Autodesk Inventor part; units mm, degrees
ref_plane "YZ Plane" through (0, 0, 0) normal (1, 0, 0) x (0, 1, 0)
ref_plane "XZ Plane" through (0, 0, 0) normal (0, 1, 0) x (-1, 0, 0)
ref_plane "XY Plane" through (0, 0, 0) normal (0, 0, 1) x (1, 0, 0)
sketch "Sketch1" plane through (0, 0, 0) normal (0, 1, 0) x (-1, 0, 0)
  line L0 (-12.7, -12.7) -> (12.7, -12.7)
  line L1 (12.7, -12.7) -> (12.7, 12.7)
  line L2 (12.7, 12.7) -> (-12.7, 12.7)
  line L3 (-12.7, 12.7) -> (-12.7, -12.7)
  line L4 (-12.7, -12.7) -> (12.7, 12.7) construction
  line L5 (12.7, -12.7) -> (-12.7, 12.7) construction
  line L6 (9.525, 9.525) -> (9.525, -9.525)
  line L7 (9.525, -9.525) -> (-9.525, -9.525)
  line L8 (-9.525, -9.525) -> (-9.525, 9.525)
  line L9 (-9.525, 9.525) -> (9.525, 9.525)
  point P0 (0, 0)
  dimension "d0" = 25.4
  dimension "d1" = 25.4
  dimension "d2" = 3.175
extrude "Extrusion1" add sketch "Sketch1" along normal mid plane 711.2
sketch "Sketch2" plane through (-12.7, 355.6, 12.7) normal (0, 0, 1) x (1, 0, 0)
  line L0 (0, 0) -> (25.4, 0)
  line L1 (0, 0) -> (25.4, -25.4)
  line L2 (25.4, -711.2) -> (25.4, 0)
  circle A0 centre (12.7, -31.75) radius 3.2512
  circle A1 centre (12.7, -50.8) radius 3.2512
  line L3 (0, -711.2) -> (0, 0)
  line L4 (0, -355.6) -> (25.4, -355.6) construction
  line L5 (0, -711.2) -> (25.4, -711.2)
  line L6 (0, -711.2) -> (25.4, -685.8)
  circle A2 centre (12.7, -679.45) radius 3.2512
  circle A3 centre (12.7, -660.4) radius 3.2512
  circle A4 centre (12.7, -12.7) radius 3.2512
  circle A5 centre (12.7, -698.5) radius 3.2512
  point P0 (12.7, -355.6)
  point P1 (12.7, 0)
  point P2 (12.7, -711.2)
  point P3 (14.9989, -14.9989)
  point P4 (10.4011, -10.4011)
  point P5 (14.9989, -696.2011)
  point P6 (10.4011, -700.7989)
  dimension "d5" = 25.4
  dimension "d6" = 6.5024
  dimension "d7" = 31.75
  dimension "d8" = 19.05
extrude "Extrusion2" cut sketch "Sketch2" against normal blind 711.2 contours L0 L2 L1 A4 | A4 L1 | L1 A4 | L6 A5 L2 L5 | A5 L6 | L6 A5 | A0 | A1 | A2 | A3
sketch "Sketch4" plane through (-12.7, -355.6, 12.7) normal (0, 0, 1) x (1, 0, 0)
  line L0 (0, 0) -> (0, 711.2) construction
  line L1 (0, 355.6) -> (25.4, 355.6) construction
  line L2 (25.4, 25.4) -> (25.4, 685.8) construction
  circle A0 centre (12.7, 171.45) radius 3.2512
  circle A1 centre (12.7, 539.75) radius 3.2512
  point P0 (12.7, 355.6)
  dimension "d23" = 6.5024
  dimension "d24" = 6.5024
  dimension "d25" = 184.15
extrude "Extrusion4" cut sketch "Sketch4" against normal blind 25.4
sketch "Sketch5" plane through (12.7, -330.2, -12.7) normal (1, 0, 0) x (0, 0, -1)
  line L0 (0, 685.8) -> (0, -25.4)
  line L1 (0, 330.2) -> (-25.4, 330.2)
  line L2 (-25.4, 0) -> (-25.4, 660.4)
  circle A0 centre (-12.7, 279.4) radius 3.2512
  circle A1 centre (-12.7, 381) radius 3.2512
  line L3 (-25.4, -25.4) -> (0, -25.4)
  point P0 (-12.7, 330.2)
  point P1 (-12.7, 330.2)
  dimension "d26" = 6.5024
  dimension "d27" = 304.8
extrude "Extrusion5" [suppressed]
sketch "Sketch9" plane through (-12.7, -355.6, 12.7) normal (0, 0, 1) x (1, 0, 0)
  line L0 (0, 0) -> (0, 711.2)
  line L1 (0, 355.6) -> (25.4, 355.6)
  line L2 (25.4, 25.4) -> (25.4, 685.8) construction
  line L3 (12.7, 247.65) -> (12.7, 463.55) construction
  circle A0 centre (12.7, 463.55) radius 3.2512
  circle A1 centre (12.7, 247.65) radius 3.2512
  point P0 (12.7, 355.6)
  point P1 (12.7, 355.6)
  dimension "d36" = 215.9
  dimension "d37" = 6.5024
extrude "Extrusion6" cut sketch "Sketch9" against normal blind 25.4
properties part number "STRU_003_BilletPole_28in_Angled_Unique" material "Aluminum 6061"
Model file for the job. Use its own axes, mm. A direction names the side the tool comes from. Give positions to 0.01 mm unless a question says otherwise; leave off trailing zeros. Write each loop counter-clockwise with the first axis right and the second up, starting at its lowest first coordinate (ties: lowest second). Pieces come first, ordered by that corner, then holes. Notation, with made-up numbers: (-7, -18.75) -> (-1, -18.75) arc R27 cw to (-1, -0.75) -> close; hole circle Ø2 at (-37, 45). An arc over 180 degrees is marked (long way). Use CSV: the item, a comma, the result in double quotes. Start each with the question number.
1) Tool access for faces 5 (the flat face through (12.7, -5, 0)), 6 (the flat face through (0, -5, 9.525)): list every direction of +Z, -Z, +X, -X, +Y, -Y with a clear straight run to the whole face (end or side of a thin tool).
2) Two-plate mould, pull along Z, no slides. Class faces 1 (the flat face through (0, -5, -12.7)), 2 (the flat face through (-9.525, -5, 0)), 3 (the flat face through (0, -5, 12.7)), 4 (the flat face through (0, -5, -9.525)): released by +Z, released by -Z, zero draft, split by the parting line, or undercut.
3) Pin check, flat tips, straight feed: P1, Ø4, axis at x = 0, y = 107.95, coming from the -Z side; P2, Ø10.5, axis at x = 0, y = -323.85, coming from the +Z side. Stop position of each tip, or through.
4) Cut at A-A on y = 213.5. List the corners of the cut face in (x, z) (3 decimals).
5) Drill centre lines: L1, parallel to Z at x = 7, y = -228 (3 decimals); L2, parallel to X at y = -304.8, z = 11.3. Where is each one in solid material? Low to high.
Final values:
1,face 5,"+Z, -Z, +X, +Y, -Y"
1,face 6,"+Y, -Y"
2,face 1,"released by -Z"
2,face 2,"undercut"
2,face 3,"released by +Z"
2,face 4,"undercut"
3,P1,"passes through"
3,P2,"stops at z = 12.7"
4,outline,"(-12.7, -12.7) -> (12.7, -12.7) -> (12.7, 12.7) -> (-12.7, 12.7) -> close; hole (-9.525, -9.525) -> (9.525, -9.525) -> (9.525, 9.525) -> (-9.525, 9.525) -> close"
5,L1,"z = -12.7 to -9.525, 9.525 to 12.7"
5,L2,"x = -12.7 to -3.25, 3.25 to 12.7"
